from build123d import *

# Parameters (mm, degrees)
SKETCH2_R           = 37.5
BOSS_EXTRUDE1_DEPTH = 2
CIRPATTERN1_COUNT   = 6
SKETCH6_R           = 12.5
CUT_EXTRUDE1_DEPTH  = 1
SKETCH7_R           = 10
BOSS_EXTRUDE2_DEPTH = 9
SKETCH8_R           = 5
CUT_EXTRUDE2_DEPTH  = 8


with BuildPart() as part:
    # Sketch2 → Boss-Extrude1 (new body)
    with BuildSketch(Plane(origin=(0, 0, 0), x_dir=(1, 0, 0), z_dir=(0, 1, 0))):
        with Locations(Location((0, 0, 0), (0, 0, 270))):
            Circle(SKETCH2_R)
    extrude(amount=BOSS_EXTRUDE1_DEPTH)

    # Sketch3 for Loft1 → Loft1 section 0
    with BuildSketch(Plane(origin=(0, 2, 0), x_dir=(1, 0, 0), z_dir=(0, 1, 0))):
        with BuildLine():
            Line((0, -15), (0, -27.124270964))
            # circular arc as an exact rational Bezier (weights 1, cos(half-angle), 1)
            Bezier((0, -27.124270964), (2.164566304, -27.124270964), (4.301737718, -26.780984447), weights=[1, 0.996830963, 1])
            Line((4.301737718, -26.780984447), (6.447780139, -13.543490366))
            Bezier((6.447780139, -13.543490366), (3.388397874, -15), (0, -15), weights=[1, 0.975422821, 1])
        make_face()
    # Sketch4 for Loft1 → Loft1 section 1
    with BuildSketch(Plane(origin=(0, 8, 0), x_dir=(1, 0, 0), z_dir=(0, 1, 0))):
        with BuildLine():
            Line((0.4, -15.012151174), (0.4, -27.112269684))
            Bezier((0.4, -27.112269684), (0.86490704, -27.099253481), (1.32975035, -27.114375462), weights=[1, 0.999542352, 1])
            Line((1.32975035, -27.114375462), (1.32975035, -14.94692609))
            Line((1.32975035, -14.94692609), (0.4, -15.012151174))
        make_face()
    loft1 = loft()

    # CirPattern1: Loft1 ×6 about axis
    cirpattern1_axis = Axis((0, -1000, 0), (0, 1, 0))
    for i in range(1, CIRPATTERN1_COUNT):
        add(loft1.rotate(cirpattern1_axis, i * 360 / CIRPATTERN1_COUNT))

    # Sketch6 → Cut-Extrude1 (cut)
    with BuildSketch(Plane(origin=(0, 2, 0), x_dir=(1, 0, 0), z_dir=(0, 1, 0))):
        with Locations(Location((0, 0, 0), (0, 0, 270))):
            Circle(SKETCH6_R)
    extrude(amount=-CUT_EXTRUDE1_DEPTH, mode=Mode.SUBTRACT)

    # Sketch7 → Boss-Extrude2 (add)
    with BuildSketch(Plane(origin=(0, 1, 0), x_dir=(1, 0, 0), z_dir=(0, 1, 0))):
        with Locations(Location((0, 0, 0), (0, 0, 270))):
            Circle(SKETCH7_R)
    extrude(amount=BOSS_EXTRUDE2_DEPTH)

    # Sketch8 → Cut-Extrude2 (cut)
    with BuildSketch(Plane.XZ):
        with Locations(Location((0, 0, 0), (0, 0, 270))):
            Circle(SKETCH8_R)
    extrude(amount=-CUT_EXTRUDE2_DEPTH, mode=Mode.SUBTRACT)


solid = part.part
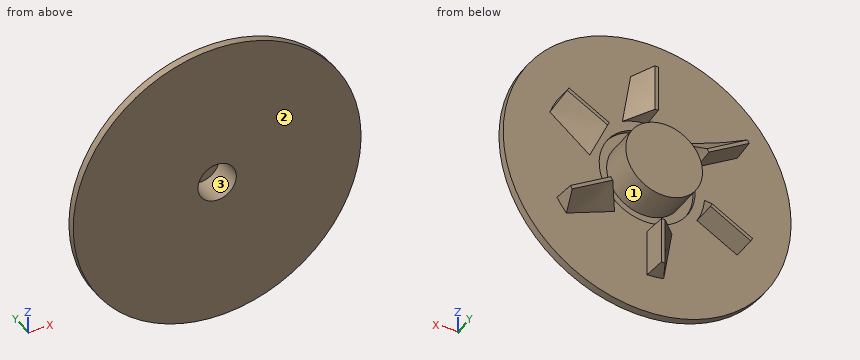
The listing builds one solid part. Answer for the finished solid, in the listing's coordinates (mm). Face numbers are marked on the shaded views. Give positions to 0.01 mm unless a question says otherwise; leave off trailing zeros. Write each loop counter-clockwise with the first axis right and the second up, starting at its lowest first coordinate (ties: lowest second). Pieces come first, ordered by that corner, then holes.
1) For a pull along X with two mould halves and no side action, classify the marked faces 1, 2 and 3 as pulls with the +X half, pulls with the -X half, needs draft (parallel to the pull), parting line crosses it, or undercut.
2) Section B-B (y = 3.75) is taken. Count the separate pieces of the cut face and the enclosed holes in it, and give its area (3 significant figures).
3) Section C-C (x = -7.5) is taken. Write down the section's boundary in (y, z).
4) Section A-A (z = 0) is taken. Write down the section's boundary in (x, y).
5) Given P1, Ø2, axis at y = 5, z = 25.5, coming from the +X side; P2, Ø6, axis at x = -13.5, y = 1, coming from the +Z side; P3, Ø1, axis at y = 4, z = 7, coming from the -X side; P4, Ø4, axis at x = 1, z = -16, coming from the -Y side, each flat-ended and moving along its own axis, determine where each tip first touches the part or whether it passes through.
6) Section D-D (y = 9) is taken. Write down the section's boundary in (x, z).
7) Find the intervals of material crossed by L1, parallel to X at y = 1.45, z = 0; L2, parallel to X at y = 4.25, z = 0; L3, parallel to Z at x = 1, y = 7.25, in increasing order.
Response:
1. face 1: undercut
1. face 2: needs draft
1. face 3: undercut
2. separate pieces: 7
2. enclosed holes: 1
2. area: 535 mm2
3. outline: (0, -36.74) - (2, -36.74) - (2, -10) - (1, -10) - (1, -6.61) - (10, -6.61) - (10, 6.61) - (1, 6.61) - (1, 10) - (2, 10) - (2, 36.74) - (0, 36.74) - close
4. outline: (-37.5, 0) - (-5, 0) - (-5, 8) - (5, 8) - (5, 0) - (37.5, 0) - (37.5, 2) - (12.5, 2) - (12.5, 1) - (10, 1) - (10, 10) - (-10, 10) - (-10, 1) - (-12.5, 1) - (-12.5, 2) - (-37.5, 2) - close
5. P1: stops at x = 3.48
5. P2: stops at z = 36
5. P3: stops at x = -7.6
5. P4: stops at y = 0
6. outline: circle Ø20 at (0, 0)
7. L1: x = -37.5 to -12.5, -10 to -5, 5 to 10, 12.5 to 37.5
7. L2: x = -10 to -5, 5 to 10
7. L3: z = -9.95 to -4.9, 4.9 to 9.95, 14.96 to 27.1
